Verification items for the finished model (mm, model axes). Face numbers are marked on the shaded views. Give positions to 0.01 mm unless a question says otherwise; leave off trailing zeros. Write each loop counter-clockwise with the first axis right and the second up, starting at its lowest first coordinate (ties: lowest second). Pieces come first, ordered by that corner, then holes. Notation, with made-up numbers: (10, -26) -> (37, -26) arc R14 ccw to (37, -5) -> close; hole circle Ø1 at (-4.75, 1). An arc over 180 degrees is marked (long way). Use CSV: the item, a comma, the result in double quotes. Start each with the question number.
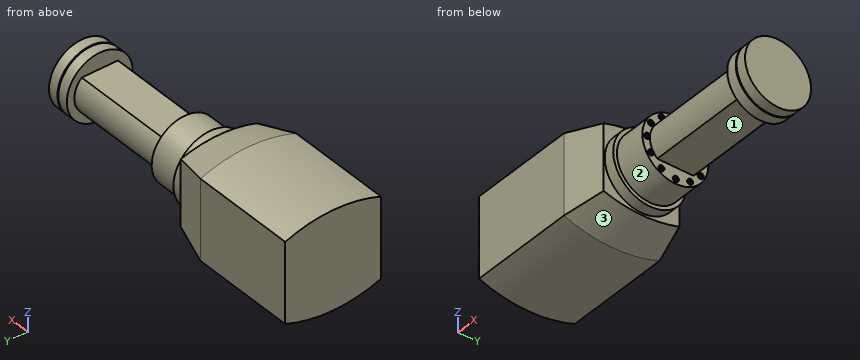
Autodesk Fusion 360 part; units mm, degrees
sketch "Sketch1" plane through (0, 0, 0) normal (1, 0, 0) x (0, 0, -1)
  line L0 (0, 0) -> (0, 45)
  line L1 (0, 0) -> (0, -45)
  line L2 (0, 45) -> (37.5, 45)
  line L3 (0, 45) -> (-37.5, 45)
  line L4 (0, -45) -> (37.5, -45)
  line L5 (0, -45) -> (-37.5, -45)
  arc A0 (-37.5, 45) -> (-37.5, -45) centre (79.119, 0) ccw
  arc A1 (37.5, -45) -> (37.5, 45) centre (-79.119, 0) ccw
  dimension "d1" = 45
  dimension "d2" = 45
  dimension "d3" = 37.5
  dimension "d4" = 37.5
  dimension "d5" = 37.5
  dimension "d6" = 37.5
  dimension "d8" = 125
extrude "Extrude1" add sketch "Sketch1" along normal blind 100
extrude "Extrude2" add 1 faces at (100, -15.2642, -14.2806) along direction (1, 0, 0) blind 35 draft -15
sketch "Sketch2" plane through (135, 0, 0) normal (1, 0, 0) x (0, 0, -1)
  line L0 (-30.8786, -35.6218) -> (30.8786, -35.6218)
  arc A0 (30.8786, -35.6218) -> (30.8786, 35.6218) centre (-79.119, 0) ccw
  line L1 (30.8786, 35.6218) -> (-30.8786, 35.6218)
  arc A1 (-30.8786, 35.6218) -> (-30.8786, -35.6218) centre (79.119, 0) ccw
  circle A2 centre (0, 0) radius 34.5
  dimension "d13" = 69
extrude "Extrude3" add sketch "Sketch2" along normal blind 10 contours A2
sketch "Sketch3" plane through (145, 0, 0) normal (1, 0, 0) x (0, 0, -1)
  circle A0 centre (0, 0) radius 34.5
  circle A1 centre (0, 0) radius 31
  dimension "d16" = 62
extrude "Extrude4" add sketch "Sketch3" along normal blind 30 contours A1
sketch "Sketch4" plane through (175, 0, 0) normal (1, 0, 0) x (0, 0, -1)
  circle A0 centre (0, 0) radius 31
  line L0 (0, 0) -> (27, 0)
  circle A1 centre (27, 0) radius 2.5
  circle A2 centre (27, 0) radius 1.5
  dimension "d19" = 27
  dimension "d20" = 5
  dimension "d21" = -1
extrude "Extrude5" add sketch "Sketch4" along normal blind 1 contours A1
pattern_circular "C-Pattern1" count 12 over 360 about axis through (175, 0, 0) along (1, 0, 0) of "Extrude5"
sketch "Sketch5" plane through (175, 0, 0) normal (1, 0, 0) x (0, 0, -1)
  circle A0 centre (27, 0) radius 2.5
  circle A1 centre (0, 0) radius 31
  circle A2 centre (23.3827, 13.5) radius 2.5
  circle A3 centre (13.5, 23.3827) radius 2.5
  circle A4 centre (0, 27) radius 2.5
  circle A5 centre (-13.5, 23.3827) radius 2.5
  circle A6 centre (-23.3827, 13.5) radius 2.5
  circle A7 centre (-27, 0) radius 2.5
  circle A8 centre (-23.3827, -13.5) radius 2.5
  circle A9 centre (-13.5, -23.3827) radius 2.5
  circle A10 centre (0, -27) radius 2.5
  circle A11 centre (13.5, -23.3827) radius 2.5
  circle A12 centre (23.3827, -13.5) radius 2.5
  line L0 (0, 0) -> (16, 0)
  line L1 (16, 0) -> (16, 17)
  line L2 (16, 0) -> (16, -17)
  line L3 (0, 0) -> (0, -8.0593)
  line L4 (-16, 0) -> (-16, 17)
  line L5 (-16, 0) -> (-16, -17)
  arc A13 (16, 17) -> (-16, 17) centre (0, 1.9003) ccw
  arc A14 (-16, -17) -> (16, -17) centre (0, -1.9003) ccw
  dimension "d26" = 16
  dimension "d27" = 17
  dimension "d28" = 17
  dimension "d29" = 22
extrude "Extrude6" add sketch "Sketch5" along normal blind 100 contours L1 L2 L4 L5 A13 A14
sketch "Sketch6" plane through (275, 0, 0) normal (1, 0, 0) x (0, 0, -1)
  line L0 (-16, 17) -> (-16, -17)
  arc A0 (-16, -17) -> (16, -17) centre (0, -1.9003) ccw
  line L1 (16, -17) -> (16, 17)
  arc A1 (16, 17) -> (-16, 17) centre (0, 1.9003) ccw
  circle A2 centre (0, 0) radius 31
  circle A3 centre (0, 0) radius 30
  dimension "d32" = 62
  dimension "d35" = -1
extrude "Extrude7" add sketch "Sketch6" along normal blind 10 contours L0 A0 L1 A1 | A2 | A3
sketch "Sketch7" plane through (285, 0, 0) normal (1, 0, 0) x (0, 0, -1)
  circle A0 centre (0, 0) radius 31
  circle A1 centre (0, 0) radius 30
  dimension "d36" = -1
extrude "Extrude8" add sketch "Sketch7" along normal blind 1 contours A1
sketch "Sketch8" plane through (286, 0, 0) normal (1, 0, 0) x (0, 0, -1)
  circle A0 centre (0, 0) radius 30
  circle A1 centre (0, 0) radius 31
  dimension "d39" = 62
extrude "Extrude9" add sketch "Sketch8" along normal blind 10 contours A0 | A1
(1) Section check C-C on x = 107. Record the cut outline in (y, z).
(2) Go/stop test with flat-tipped pins: pin 1 (6 mm diameter, centred on x = 111.5, z = -35, fed in from -Y); pin 2 (17 mm diameter, centred on x = 217.5, y = 3, fed in from +Z); pin 3 (8 mm diameter, centred on y = 19, z = -33, fed in from +X). Record where each tip stops, or that it passes through.
(3) Section check A-A on x = 164. Record the cut outline in (y, z), then the cut area to 3 significant figures.
(4) Thickness scan on line 1 (Z direction, x = 175.2, y = -13.5); line 2 (X direction, y = 0, z = -21); line 3 (Y direction, x = 175.8, z = -13.5). Record the ranges inside material, lowest first. Write a range as from..to.
(5) Section check B-B on x = 217. Record the cut outline in (y, z).
(6) Draft check along X on the marked faces 1, 2 and 3. Enter one of: released by +X, released by -X, zero draft, split by the parting line, or undercut.
Data:
1,outline,"(-43.12, -36.21) arc R123.12 ccw to (43.12, -36.21) -> (43.12, 36.21) arc R123.12 ccw to (-43.12, 36.21) -> close"
2,pin 1,"stops at y = -42.72"
2,pin 2,"stops at z = 16"
2,pin 3,"stops at x = 145"
3,outline,"circle Ø62 at (0, 0)"
3,area,"3,020 mm2"
4,line 1,"z = -25.88..-24.88, -21.88..-20.88, -16..16, 20.88..21.88, 24.88..25.88"
4,line 2,"x = 0..175, 275..296"
4,line 3,"y = -25.88..-24.88, -21.88..-20.88, -19.27..19.27, 20.88..21.88, 24.88..25.88"
5,outline,"(-17, -16) -> (17, -16) arc R22 ccw to (17, 16) -> (-17, 16) arc R22 ccw to start"
6,face 1,"undercut"
6,face 2,"zero draft"
6,face 3,"released by +X"
